Can you work these out from the drawing? Everything is in mm from the part's minimum corner. A direction names the side the tool comes from. Round coordinates to 2 decimals unless told otherwise and drop trailing zeros. Loops run counter-clockwise (first coordinate to the right, second up) from the corner with the lowest first, then second, coordinate; pieces in that order, holes last. Notation, with made-up numbers: (-13, 25.5) -> (26, 25.5) arc R14 ccw to (26, 36.5) -> close; hole circle Ø4 at (35.5, 40.5). An arc over 180 degrees is marked (long way). One line per item, written item: value.
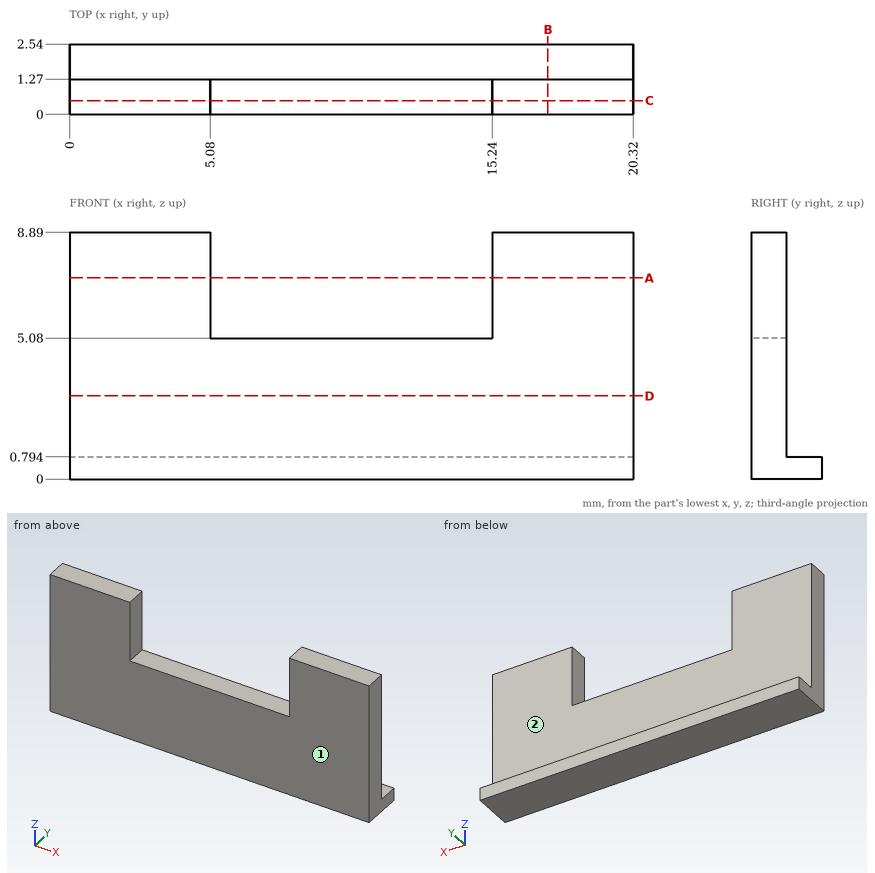
(1) If we section it at C-C, the plane y = 0.5: Please give me the cut outline in (x, z), then the cut area to 3 significant figures.
Recorded:
outline: (0, 0) -> (20.32, 0) -> (20.32, 8.89) -> (15.24, 8.89) -> (15.24, 5.08) -> (5.08, 5.08) -> (5.08, 8.89) -> (0, 8.89) -> close
area: 142 mm²
(2) If I drill on L1, parallel to X at y = 0.65, z = 6; L2, parallel to Y at x = 3.25, z = 3.25; L3, parallel to Z at x = 10, y = 1.5, over which ranges is the centre line in solid material (lowest first)?
Recorded:
L1: 0 to 5.08, 15.24 to 20.32
L2: 0 to 1.27
L3: 0 to 0.79
(3) If we section it at A-A, the plane z = 7.25: Please give me the cut outline in (x, y).
Recorded:
outline: (0, 0) -> (5.08, 0) -> (5.08, 1.27) -> (0, 1.27) -> close; (15.24, 0) -> (20.32, 0) -> (20.32, 1.27) -> (15.24, 1.27) -> close
(4) If we section it at B-B, the plane x = 17.25: Please give me the cut outline in (y, z), then the cut area to 3 significant figures.
Recorded:
outline: (0, 0) -> (2.54, 0) -> (2.54, 0.79) -> (1.27, 0.79) -> (1.27, 8.89) -> (0, 8.89) -> close
area: 12.3 mm²
(5) I'm going to push flat-ended pins straight in: pin 1 Ø3 at (x, z) = (10, 4.5) entering from -Y; pin 2 Ø4 at (x, z) = (13, 5) entering from +Y; pin 3 Ø1 at (x, y) = (8, 0.5) entering from +Z. Where does each tip first touch, or does it pass through?
Recorded:
pin 1: y = 0
pin 2: y = 1.27
pin 3: z = 5.08
(6) For the marked faces 1 and 2, which set-ups out of +Z, -Z, +X, -X, +Y, -Y let a thin tool reach every point of the face, with its end or its side?
Recorded:
face 1: +Z, -Z, +X, -X, -Y
face 2: +Z, +X, -X, +Y
(7) If we section it at D-D, the plane z = 3: Please give me the cut outline in (x, y), then the cut area to 3 significant figures.
Recorded:
outline: (0, 0) -> (20.32, 0) -> (20.32, 1.27) -> (0, 1.27) -> close
area: 25.8 mm²
